Model file for the job. Use its own axes, mm. Coordinates: 2 decimals unless noted, no trailing zeros. Loops run counter-clockwise (first coordinate to the right, second up) from the corner with the lowest first, then second, coordinate; pieces in that order, holes last. Notation, with made-up numbers: (26, -16) - (38, -16) arc R16 cw to (38, 6) - close; hole circle Ø5 at (-35, 13). An arc over 180 degrees is marked (long way). Write each question's results on one line, items separated by ' | '. Start each with the question number.
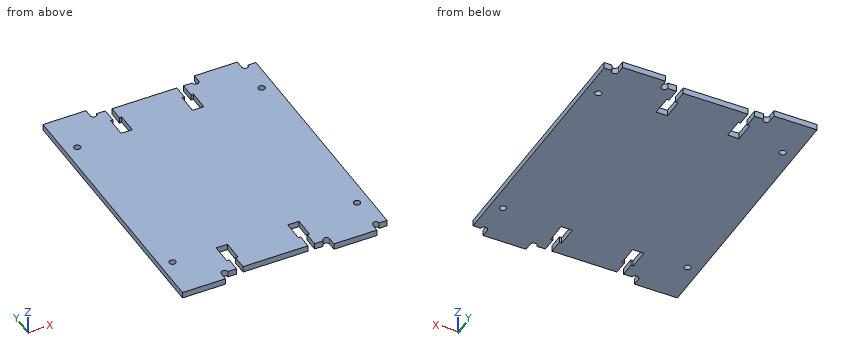
```python
from build123d import *

# Parameters (mm, degrees)
MODEL_R             = 1.6
BOSS_EXTRUDE1_DEPTH = 3
SKETCH2_R           = 1.59
CUT_EXTRUDE1_DEPTH  = 135.365174059


with BuildPart() as part:
    # Model → Boss-Extrude1 (new body)
    with BuildSketch(Plane.XY):
        Polygon((110, -66), (110, -62), (117, -62), (117, 62), (110, 62), (110, 66), (89, 66), (89, 62), (81.6, 62), (81.6, 55), (82.75, 55), (82.75, 45), (77.25, 45), (77.25, 55), (78.4, 55), (78.4, 62), (46.65, 62), (46.65, 55), (47.8, 55), (47.8, 45), (42.3, 45), (42.3, 55), (43.45, 55), (43.45, 62), (36, 62), (36, 66), (15, 66), (15, -66), (36, -66), (36, -62), (43.45, -62), (43.45, -55), (42.3, -55), (42.3, -45), (47.8, -45), (47.8, -55), (46.65, -55), (46.65, -62), (78.4, -62), (78.4, -55), (77.25, -55), (77.25, -45), (82.75, -45), (82.75, -55), (81.6, -55), (81.6, -62), (89, -62), (89, -66), align=None)
        with Locations((111.085, -45.085)):
            Circle(MODEL_R, mode=Mode.SUBTRACT)
        with Locations((111.085, 45.085)):
            Circle(MODEL_R, mode=Mode.SUBTRACT)
        with Locations((20.915, 45.085)):
            Circle(MODEL_R, mode=Mode.SUBTRACT)
        with Locations((20.915, -45.085)):
            Circle(MODEL_R, mode=Mode.SUBTRACT)
    extrude(amount=BOSS_EXTRUDE1_DEPTH)

    # Sketch2 → Cut-Extrude1 (cut, through all)
    with BuildSketch(Plane.XY.offset(3)):
        with Locations((37.59, 62)):
            Circle(SKETCH2_R)
        with Locations((87.41, 62)):
            Circle(SKETCH2_R)
        with Locations((37.59, -62)):
            Circle(SKETCH2_R)
        with Locations((87.41, -62)):
            Circle(SKETCH2_R)
        with Locations((111.59, -62)):
            Circle(SKETCH2_R)
        with Locations((111.59, 62)):
            Circle(SKETCH2_R)
    extrude(amount=-CUT_EXTRUDE1_DEPTH, mode=Mode.SUBTRACT)


solid = part.part
```
Q1. Cut at B-B (z = 0.7). State how many separate pieces and enclosed holes the cut face has, and give its area (3 significant figures).
Q2. Drill centre lines: L1, parallel to X at y = 47, z = 0.4; L2, parallel to Y at x = 111, z = 2.65; L3, parallel to Y at x = 61.5, z = 2.65. Where is each one in solid material? Low to high. Write a range as from..to.
Q3. Pin check, flat tips, straight feed: pin 1 (1.3 mm diameter, centred on x = 82, z = 2, fed in from +Y); pin 2 (0.9 mm diameter, centred on y = -63, z = 1.5, fed in from +X); pin 3 (1.3 mm diameter, centred on x = 77.5, z = 2, fed in from -Y). Stop position of each tip, or through.
Q4. Cut at C-C (x = 87.41). List the corners of the cut face in (y, z).
Q5. Cut at A-A (x = 54). List the corners of the cut face in (y, z).
Check result:
1) separate pieces: 1 | enclosed holes: 4 | area: 12,600 mm²
2) L1: 15..42.3, 47.8..77.25, 82.75..117 | L2: -60.52..-46.68, -43.49..43.49, 46.68..60.52 | L3: -62..62
3) pin 1: y = 62 | pin 2: x = 110 | pin 3: y = -62
4) outline: (-60.41, 0) - (60.41, 0) - (60.41, 3) - (-60.41, 3) - close
5) outline: (-62, 0) - (62, 0) - (62, 3) - (-62, 3) - close
